The model under review builds one solid part; all positions refer to its coordinate system, in mm. A direction names the side the tool comes from. Give positions to 0.01 mm unless a question says otherwise; leave off trailing zeros. Loops run counter-clockwise (first coordinate to the right, second up) from the corner with the lowest first, then second, coordinate; pieces in that order, holes last. Notation, with made-up numbers: M 11,9 L 33,9 A28 ccw 33,40 Z; hole C 79,69.25 d9. An arc over 180 degrees is marked long. Put each result on its own line as item: value. Start each with the question number.
Autodesk Inventor part; units mm, degrees
ref_plane "YZ Plane" through (0, 0, 0) normal (1, 0, 0) x (0, 1, 0)
ref_plane "XZ Plane" through (0, 0, 0) normal (0, 1, 0) x (-1, 0, 0)
ref_plane "XY Plane" through (0, 0, 0) normal (0, 0, 1) x (1, 0, 0)
sketch "Sketch1" plane through (0, 0, 0) normal (0, 1, 0) x (-1, 0, 0)
  line L0 (-94, 28.5) -> (94, 28.5) construction
  line L1 (94, 28.5) -> (94, -28.5) construction
  line L2 (94, -28.5) -> (-94, -28.5) construction
  line L3 (-94, -28.5) -> (-94, 17.1863) construction
  line L4 (-94, 28.5) -> (94, -28.5) construction
  line L5 (94, 28.5) -> (-94, -28.5) construction
  arc A0 (86, -28.5) -> (96.6667, -20.9575) centre (94, -28.5) ccw
  arc A1 (96.6667, 20.9575) -> (86, 28.5) centre (94, 28.5) ccw
  arc A2 (-86, 28.5) -> (-96.6667, 20.9575) centre (-94, 28.5) ccw
  arc A3 (-96.6667, -20.9575) -> (-86, -28.5) centre (-94, -28.5) ccw
  line L6 (94, -17.1863) -> (94, 17.1863)
  line L7 (86, -28.5) -> (86, -26)
  line L8 (-86, -26) -> (-86, -28.5)
  line L9 (86, 28.5) -> (86, 26)
  line L10 (-86, 26) -> (-86, 28.5)
  circle A4 centre (13, 0) radius 10
  circle A5 centre (-13, 0) radius 10
  circle A6 centre (49, 0) radius 10
  circle A7 centre (75, 0) radius 10
  circle A8 centre (-49, 0) radius 10
  circle A9 centre (-75, 0) radius 10
  circle A10 centre (0, -16.75) radius 1.9
  circle A11 centre (0, 16.75) radius 1.9
  circle A12 centre (31, 16.75) radius 1.9
  circle A13 centre (-31, 16.75) radius 1.9
  arc A14 (-5.8683, -18) -> (5.8683, -18) centre (0, -16.75) ccw
  arc A15 (5.8683, 18) -> (-5.8683, 18) centre (0, 16.75) ccw
  arc A16 (36.8683, 18) -> (25.1317, 18) centre (31, 16.75) ccw
  arc A17 (-25.1317, 18) -> (-36.8683, 18) centre (-31, 16.75) ccw
  line L11 (78, -18) -> (61, -18)
  line L12 (-5.8683, -18) -> (-42.5, -18)
  line L13 (78, 18) -> (36.8683, 18)
  line L14 (25.1317, 18) -> (5.8683, 18)
  line L15 (-5.8683, 18) -> (-25.1317, 18)
  line L16 (-36.8683, 18) -> (-78, 18)
  arc A18 (86, -26) -> (78, -18) centre (78, -26) ccw
  arc A19 (78, 18) -> (86, 26) centre (78, 26) ccw
  arc A20 (-86, 26) -> (-78, 18) centre (-78, 26) ccw
  arc A21 (-78, -18) -> (-86, -26) centre (-78, -26) ccw
  arc A22 (94, -17.1863) -> (96.6667, -20.9575) centre (98, -17.1863) ccw
  arc A23 (96.6667, 20.9575) -> (94, 17.1863) centre (98, 17.1863) ccw
  arc A24 (-96.6667, -20.9575) -> (-94, -17.1863) centre (-98, -17.1863) ccw
  arc A25 (-94, 17.1863) -> (-96.6667, 20.9575) centre (-98, 17.1863) ccw
  circle A26 centre (94, -28.5) radius 1.6
  circle A27 centre (94, 28.5) radius 1.6
  circle A28 centre (-94, 28.5) radius 1.6
  circle A29 centre (-94, -28.5) radius 1.6
  line L17 (-94, -17.1863) -> (-94, 17.1863)
  line L18 (57, -22) -> (57, -29.5)
  line L19 (55, -31.5) -> (45, -31.5)
  line L20 (43, -29.5) -> (43, -22)
  line L21 (-46.5, -22) -> (-46.5, -29.5)
  line L22 (-48.5, -31.5) -> (-56.5, -31.5)
  line L23 (-58.5, -29.5) -> (-58.5, -22)
  line L24 (39, -18) -> (5.8683, -18)
  line L25 (-62.5, -18) -> (-78, -18)
  arc A30 (55, -31.5) -> (57, -29.5) centre (55, -29.5) ccw
  arc A31 (43, -29.5) -> (45, -31.5) centre (45, -29.5) ccw
  arc A32 (-48.5, -31.5) -> (-46.5, -29.5) centre (-48.5, -29.5) ccw
  arc A33 (-58.5, -29.5) -> (-56.5, -31.5) centre (-56.5, -29.5) ccw
  arc A34 (61, -18) -> (57, -22) centre (61, -22) ccw
  arc A35 (43, -22) -> (39, -18) centre (39, -22) ccw
  arc A36 (-42.5, -18) -> (-46.5, -22) centre (-42.5, -22) ccw
  arc A37 (-58.5, -22) -> (-62.5, -18) centre (-62.5, -22) ccw
  point P0 (0, 0)
  point P1 (94, 20.5)
  point P2 (-94, -20.5)
  point P3 (94, -20.5)
  point P4 (0, 0)
  point P5 (0, 0)
  point P6 (50, -31.5)
  point P7 (-52.5, -31.5)
  point P8 (57, -31.5)
  point P9 (43, -31.5)
  point P10 (43, -18)
  point P11 (-46.5, -31.5)
  point P12 (-58.5, -31.5)
  point P13 (-58.5, -18)
  point P14 (-52.5, -31.5)
  point P15 (50, -31.5)
  dimension "d0" = 188
  dimension "d1" = 57
  dimension "d2" = 20
  dimension "d3" = 26
  dimension "d4" = 13
  dimension "d5" = 36
  dimension "d6" = 26
  dimension "d7" = 36
  dimension "d8" = 26
  dimension "d9" = 8
  dimension "d10" = 16.75
  dimension "d11" = 3.8
  dimension "d12" = 16.75
  dimension "d13" = 31
  dimension "d14" = 31
  dimension "d15" = 12
  dimension "d16" = 18
  dimension "d17" = 18
  dimension "d18" = 8
  dimension "d19" = 4
  dimension "d20" = 3.2
  dimension "d23" = 50
  dimension "d24" = 52.5
  dimension "d25" = 31.5
  dimension "d26" = 14
  dimension "d27" = 12
  dimension "d28" = 2
  dimension "d29" = 4
extrude "Extrusion1" add sketch "Sketch1" along normal blind 1.5
equation "\"d6\" = d3"
equation "\"d7\" = d5"
equation "\"d8\" = d3"
properties part number "Cover"
Item 1: Consider section D-D, the plane y = 1.15. Give the number of separate pieces and of enclosed holes in the cut face, plus the area to 3 significant figures.
Item 2: To check wall thickness, follow L1, parallel to Z at x = 0, y = 0.35; L2, parallel to Z at x = 75, y = 0.9; L3, parallel to X at y = 1.25, z = -20. State the ranges of each line that lie inside material, in increasing order. Write a range as [from, to].
Item 3: Draft analysis for pull direction X (two halves, no side actions). For faces 4 (the flat face through (1, 1.5, 1)), 5 (the cylindrical face through (-83.594, 0.74, -20.281)), 6 (the cylindrical face through (83.719, 0.74, -20.406)), state which applies: +X half, -X half, draft (parallel to the pull), parting line (faces both ways), or undercut.
Item 4: Consider section B-B, the plane x = 67. Write out the cut boundary in (y, z).
Item 5: Consider section A-A, the plane z = 6. Write out the cut boundary in (x, y).
Item 6: Consider section C-C, the plane x = 0. Write out the cut boundary in (y, z), plus the area to 4 significant figures.
Item 7: Clearance check with a flat-ended pin moving along its axis: pin 1 Ø0.8 at (x, y) = (67, 1) entering from -Z. State where the tip first meets the part, or that it passes through.
Item 8: Tool access review of faces 1 (the cylindrical face through (83.594, 0.74, 20.281)), 2 (the cylindrical face through (59.703, 0.74, -19.141)), 3 (the cylindrical face through (98.8, 0.7, 34.9)): name each direction out of +Z, -Z, +X, -X, +Y, -Y from which nothing blocks a thin tool from reaching the whole face with its end or side.
Report:
1. separate pieces: 1
1. enclosed holes: 14
1. area: 6,340 mm²
2. L1: [-22.75, -18.65], [-14.85, 14.85], [18.65, 22.75]
2. L2: [-18, -10], [10, 18]
2. L3: [-95.16, -83.29], [-57.54, -42.46], [-5.04, 5.04], [45.96, 59.04], [83.29, 95.16]
3. face 4: draft
3. face 5: undercut
3. face 6: undercut
4. outline: M 0,-18 L 1.5,-18 L 1.5,-6 L 0,-6 Z; M 0,6 L 1.5,6 L 1.5,18 L 0,18 Z
5. outline: M -94,0 L -83,0 L -83,1.5 L -94,1.5 Z; M -67,0 L -57,0 L -57,1.5 L -67,1.5 Z; M -41,0 L -21,0 L -21,1.5 L -41,1.5 Z; M -5,0 L 5,0 L 5,1.5 L -5,1.5 Z; M 21,0 L 41,0 L 41,1.5 L 21,1.5 Z; M 57,0 L 67,0 L 67,1.5 L 57,1.5 Z; M 83,0 L 94,0 L 94,1.5 L 83,1.5 Z
6. outline: M 0,-22.75 L 1.5,-22.75 L 1.5,-18.65 L 0,-18.65 Z; M 0,-14.85 L 1.5,-14.85 L 1.5,14.85 L 0,14.85 Z; M 0,18.65 L 1.5,18.65 L 1.5,22.75 L 0,22.75 Z
6. area: 56.85 mm²
7. pin 1: z = -18
8. face 1: +Z, +Y, -Y
8. face 2: -Z, +Y, -Y
8. face 3: +Y, -Y
